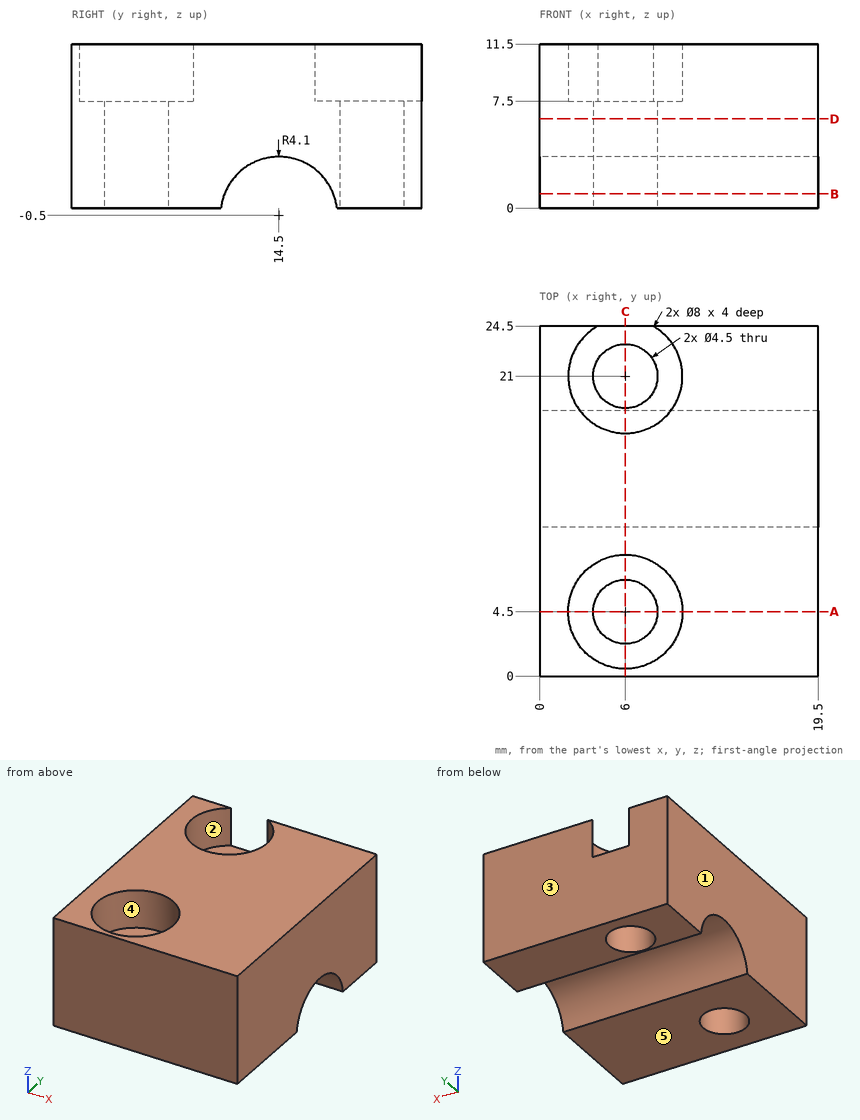
Source: three-view drawing plus pictorial views. Frame: mm from the lowest corner of the part. A direction names the side the tool comes from. Coordinates: 2 decimals unless noted, no trailing zeros. Loops run counter-clockwise (first coordinate to the right, second up) from the corner with the lowest first, then second, coordinate; pieces in that order, holes last. Notation, with made-up numbers: (12.25, 24.25) - (21.25, 24.25) arc R13 cw to (21.25, 44.25) - close; hole circle Ø2 at (24, 20). An arc over 180 degrees is marked (long way). Answer in a Markdown table with one row per item. Add a question column.
Item 1: Section query B-B on z = 1. Return the cut outline in (x, y), then the cut area to 3 significant figures.
Item 2: Mould query, pull axis X, two halves, no side actions, for the marked faces 1, 2 and 3. Classes: released by +X, released by -X, zero draft, split by the parting line, or undercut.
Item 3: Section query C-C on x = 6. Return the cut outline in (y, z), then the cut area to 3 significant figures.
Item 4: Contact query for flat-ended pins moving along their axis: P1, Ø6.5, axis at x = 6, y = 4.5, coming from the +Z side; P2, Ø3.5, axis at x = 6, y = 21, coming from the -Z side; P3, Ø4, axis at x = 15.5, y = 15, coming from the -Z side. Output: stop coordinate, or through.
Item 5: Section query A-A on y = 4.5. Return the cut outline in (x, z).
Item 6: Access query for the marked faces 4 and 5. Directions: +Z, -Z, +X, -X, +Y, -Y. A direction counts if a zero-diameter tool reaches every point of the face in a straight line with its end or side. Return the directions, or none.
Item 7: Section query D-D on z = 6.25. Return the cut outline in (x, y), then the cut area to 3 significant figures.
Item 8: Line query: line 1 along Y through (x, z) = (6, 5.75); line 2 along Y through (x, z) = (6, 8.45); line 3 along X through (y, z) = (21, 4.5). Output: solid intervals per line, ascending. Write a range as [from, to].
Recorded:
| question | item | result |
|---|---|---|
| 1 | outline | (0, 0) - (19.5, 0) - (19.5, 10.68) - (0, 10.68) - close; (0, 18.32) - (19.5, 18.32) - (19.5, 24.5) - (0, 24.5) - close; hole circle Ø4.5 at (6, 4.5); hole circle Ø4.5 at (6, 21) |
| 1 | area | 297 mm^2 |
| 2 | face 1 | released by -X |
| 2 | face 2 | undercut |
| 2 | face 3 | zero draft |
| 3 | outline | (0, 0) - (2.25, 0) - (2.25, 7.5) - (0.5, 7.5) - (0.5, 11.5) - (0, 11.5) - close; (6.75, 0) - (10.43, 0) arc R4.1 cw to (18.57, 0) - (18.75, 0) - (18.75, 7.5) - (17, 7.5) - (17, 11.5) - (8.5, 11.5) - (8.5, 7.5) - (6.75, 7.5) - close; (23.25, 0) - (24.5, 0) - (24.5, 7.5) - (23.25, 7.5) - close |
| 3 | area | 130 mm^2 |
| 4 | P1 | z = 7.5 |
| 4 | P2 | through |
| 4 | P3 | z = 2.75 |
| 5 | outline | (0, 0) - (3.75, 0) - (3.75, 7.5) - (2, 7.5) - (2, 11.5) - (0, 11.5) - close; (8.25, 0) - (19.5, 0) - (19.5, 11.5) - (10, 11.5) - (10, 7.5) - (8.25, 7.5) - close |
| 6 | face 4 | +Z |
| 6 | face 5 | -Z, +X, -X, +Y, -Y |
| 7 | outline | (0, 0) - (19.5, 0) - (19.5, 24.5) - (0, 24.5) - close; hole circle Ø4.5 at (6, 4.5); hole circle Ø4.5 at (6, 21) |
| 7 | area | 446 mm^2 |
| 8 | line 1 | [0, 2.25], [6.75, 18.75], [23.25, 24.5] |
| 8 | line 2 | [0, 0.5], [8.5, 17] |
| 8 | line 3 | [0, 3.75], [8.25, 19.5] |
